Answer from the drawing. Dimensions are ordinates in mm from the lowest x, y and z of the part. A direction names the side the tool comes from. Round coordinates to 2 decimals unless told otherwise and drop trailing zeros. Order: outer loops, then holes, each group sorted by start corner. A loop starts at its lowest first (then second) coordinate and runs counter-clockwise, first axis right, second up. Notation, with made-up numbers: (19.25, -31) -> (43.25, -31) arc R26 ccw to (43.25, -15) -> close; hole circle Ø2 at (-31, -8). An arc over 180 degrees is marked (long way). Use a Markdown table: item, result. Add a question column.
Item 1: A tool of negligible diameter and unlimited length cuts with its end or side. For the marked faces 5, 6 and 7, from which of +Z, -Z, +X, -X, +Y, -Y can it reach the whole face along a straight path? Write none if from no direction.
Item 2: Find the intervals of material crossed by L1, parallel to Z at x = 343.5, y = 571.5; L2, parallel to X at y = 750, z = 849; L3, parallel to Y at x = 211, z = 786, in increasing order. Write a range as [from, to].
Item 3: For a pull along Z with two mould halves and no side action, classify the marked faces 1, 2, 3 and 4 as +Z half, -Z half, draft (parallel to the pull), parting line (faces both ways), or undercut.
Item 4: A cutting plane is placed at D-D, the plane x = 159. Determine the outline of the cut face in (y, z), plus the area to 3 significant figures.
Item 5: A cutting plane is placed at B-B, the plane x = 73.5. Determine the outline of the cut face in (y, z), plus the area to 3 significant figures.
Item 6: A cutting plane is placed at A-A, the plane y = 483.5. Determine the outline of the cut face in (x, z), plus the area to 3 significant figures.
Item 7: Flat-ended cylindrical pins translate along their axes: P1, Ø12.5, axis at y = 17.5, z = 175, coming from the +X side; P2, Ø8, axis at x = 308.5, z = 540.5, coming from the -Y side. Find the tip coordinate at first contact, or state that the pin passes through.
Item 8: A cutting plane is placed at C-C, the plane z = 355.5. Determine the outline of the cut face in (x, y), plus the area to 3 significant figures.
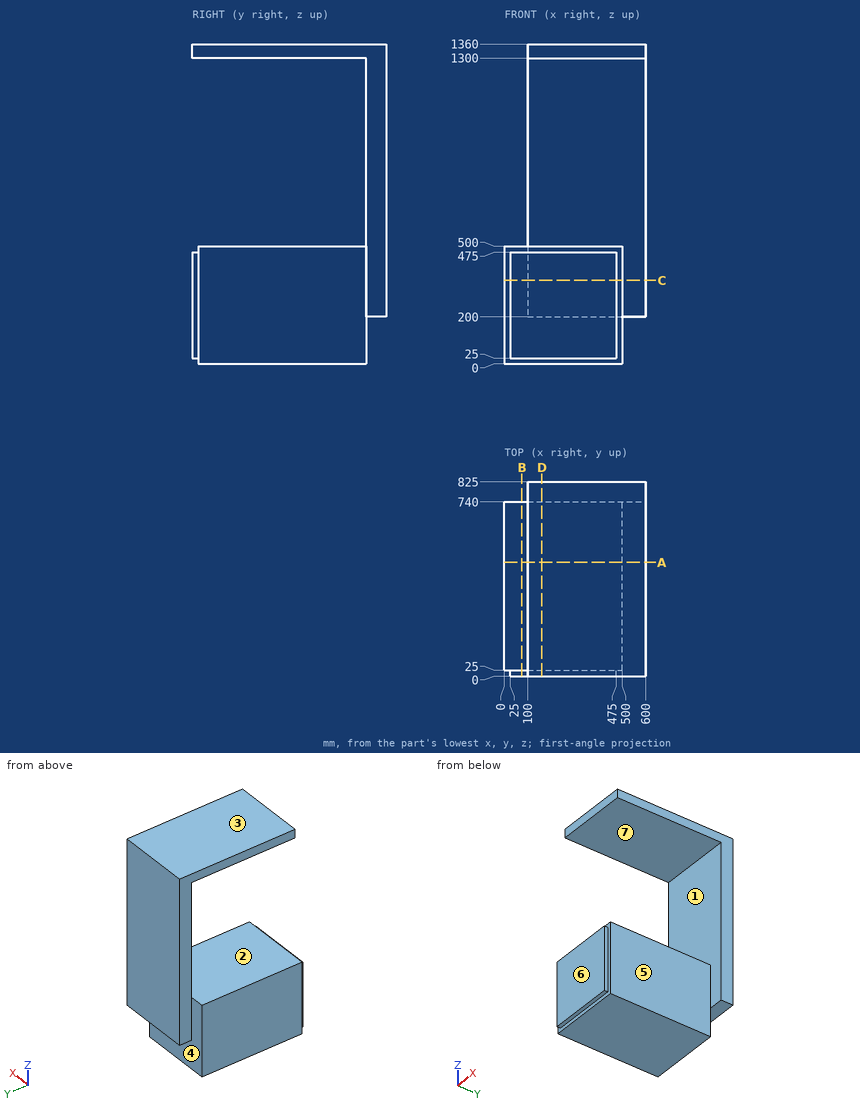
Reported:
| question | item | result |
|---|---|---|
| 1 | face 5 | -Z, +X, -Y |
| 1 | face 6 | +Z, -Z, +X, -X, -Y |
| 1 | face 7 | +X, -X, -Y |
| 2 | L1 | [0, 500], [1300, 1360] |
| 2 | L2 | [100, 600] |
| 2 | L3 | [740, 825] |
| 3 | face 1 | undercut |
| 3 | face 2 | undercut |
| 3 | face 3 | +Z half |
| 3 | face 4 | draft |
| 4 | outline | (0, 25) -> (25, 25) -> (25, 0) -> (740, 0) -> (740, 200) -> (825, 200) -> (825, 1360) -> (0, 1360) -> (0, 1300) -> (740, 1300) -> (740, 500) -> (25, 500) -> (25, 475) -> (0, 475) -> close |
| 4 | area | 512,000 mm² |
| 5 | outline | (0, 25) -> (25, 25) -> (25, 0) -> (740, 0) -> (740, 500) -> (25, 500) -> (25, 475) -> (0, 475) -> close |
| 5 | area | 369,000 mm² |
| 6 | outline | (0, 0) -> (500, 0) -> (500, 500) -> (0, 500) -> close; (100, 1300) -> (600, 1300) -> (600, 1360) -> (100, 1360) -> close |
| 6 | area | 280,000 mm² |
| 7 | P1 | x = 475 |
| 7 | P2 | y = 740 |
| 8 | outline | (0, 25) -> (25, 25) -> (25, 0) -> (475, 0) -> (475, 25) -> (500, 25) -> (500, 740) -> (600, 740) -> (600, 825) -> (100, 825) -> (100, 740) -> (0, 740) -> close |
| 8 | area | 411,000 mm² |
